Job drawing, mm, ordinate dimensions from the low corner. One solid piece. Coordinates: 2 decimals unless noted, no trailing zeros. Loops run counter-clockwise (first coordinate to the right, second up) from the corner with the lowest first, then second, coordinate; pieces in that order, holes last. Notation, with made-up numbers: (-19, -34) - (-4, -34) arc R13 ccw to (-4, -13) - close; hole circle Ø5 at (58, 73). An arc over 180 degrees is marked (long way). Use a Markdown table: item, result. Add a question column.
1) Band-saw the part on B-B (z = 76.2). Give the cut face in (x, y), plus the area to 4 significant figures.
2) Probe probe 1 along Z at (x, y) = (76.2, 6); probe 2 along X at (y, z) = (6.75, 100); probe 3 along Z at (x, y) = (128, 10) (1 decimal). List the from-to ranges inside material, lowest first. Write a range as [from, to].
3) Pull direction X, two halves, no side cores. Call the marked faces 1, 2 and 3: +X half, -X half, draft (parallel to the pull), parting line (faces both ways), or undercut.
4) Band-saw the part on A-A (x = 76.2). Give the cut face in (y, z), plus the area to 3 significant figures.
5) Band-saw the part on C-C (y = 5.75). Give the number of separate pieces and of enclosed holes in the cut face, plus the area to 3 significant figures.
6) Band-saw the part on D-D (z = 107). Give the cut face in (x, y) (1 decimal), plus the area to 3 significant figures.
7) Drop flat-ended pins along their axis: P1, Ø7, axis at x = 26.71, z = 104.78, coming from the +Y side; P2, Ø1.5, axis at x = 83, y = 7, coming from the -Z side; P3, Ø1, axis at x = 89.5, y = 8.5, coming from the -Z side; P4, Ø1.5, axis at x = 15.5, y = 2.5, coming from the +Z side (1 decimal). Give the stop position or say it passes through.
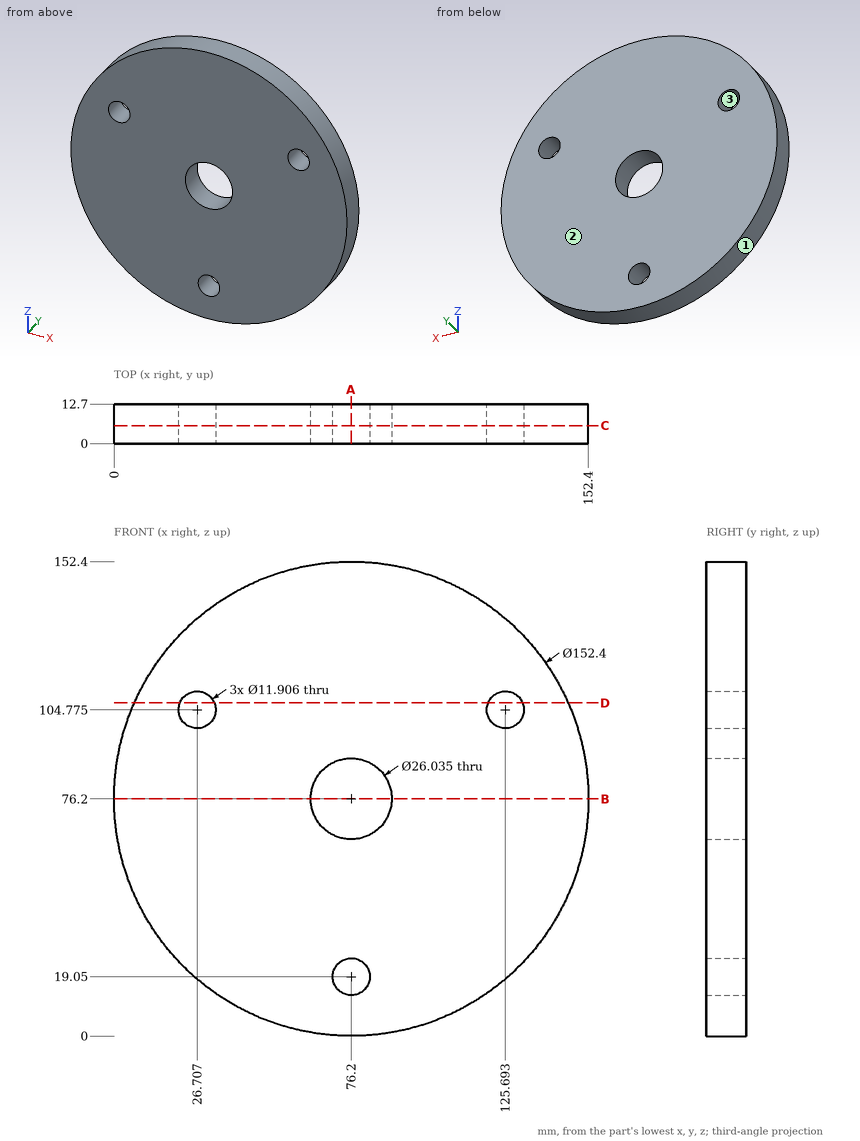
Answer block:
| question | item | result |
|---|---|---|
| 1 | outline | (0, 0) - (63.18, 0) - (63.18, 12.7) - (0, 12.7) - close; (89.22, 0) - (152.4, 0) - (152.4, 12.7) - (89.22, 12.7) - close |
| 1 | area | 1,605 mm2 |
| 2 | probe 1 | [0, 13.1], [25, 63.18], [89.22, 152.4] |
| 2 | probe 2 | [3.81, 23.15], [30.26, 122.14], [129.25, 148.59] |
| 2 | probe 3 | [20.3, 99.3], [110.3, 132.1] |
| 3 | face 1 | parting line |
| 3 | face 2 | draft |
| 3 | face 3 | undercut |
| 4 | outline | (0, 0) - (12.7, 0) - (12.7, 13.1) - (0, 13.1) - close; (0, 25) - (12.7, 25) - (12.7, 63.18) - (0, 63.18) - close; (0, 89.22) - (12.7, 89.22) - (12.7, 152.4) - (0, 152.4) - close |
| 4 | area | 1,450 mm2 |
| 5 | separate pieces | 1 |
| 5 | enclosed holes | 4 |
| 5 | area | 17,400 mm2 |
| 6 | outline | (6.5, 0) - (21.2, 0) - (21.2, 12.7) - (6.5, 12.7) - close; (32.2, 0) - (120.2, 0) - (120.2, 12.7) - (32.2, 12.7) - close; (131.2, 0) - (145.9, 0) - (145.9, 12.7) - (131.2, 12.7) - close |
| 6 | area | 1,490 mm2 |
| 7 | P1 | through |
| 7 | P2 | z = 0.24 |
| 7 | P3 | z = 1.08 |
| 7 | P4 | z = 123.2 |
